Verification items for the finished model (mm, model axes). A direction names the side the tool comes from. Give positions to 0.01 mm unless a question says otherwise; leave off trailing zeros. Write each loop counter-clockwise with the first axis right and the second up, starting at its lowest first coordinate (ties: lowest second). Pieces come first, ordered by that corner, then holes. Notation, with made-up numbers: (81, 15) - (122, 15) arc R21 ccw to (122, 51) - close; hole circle Ø10 at (85, -22). An arc over 180 degrees is marked (long way). Put each result on its own line as item: value.
from build123d import *

# Parameters (mm, degrees)
F2_R     = 2
F3_DEPTH = 12.5
F5_R     = 2
F6_DEPTH = 25


with BuildPart() as f1:
    # F0 (on Top) → F1 (revolve)
    with BuildSketch(Plane.XY):
        with BuildLine():
            Line((32.238782, 5), (-36.118835, 5))
            ThreePointArc((-36.118835, 5), (-47.25717, 4.119532), (-58.118835, 1.5))
            ThreePointArc((-58.118835, 1.5), (-59.179495, 1.06066), (-59.618835, 0))
            Line((-59.618835, 0), (-58.118835, 0))
            Line((-58.118835, 0), (-36.118835, 0))
            Line((-36.118835, 0), (32.238782, 0))
            Line((32.238782, 0), (50.381165, 0))
            ThreePointArc((50.381165, 0), (41.648166, 3.727125), (32.238782, 5))
        make_face()
    revolve(axis=Axis((-7.075977, 0, 0), (1, 0, 0)))

    # F2 (on Front) → F3 (cut, symmetric)
    with BuildSketch(Plane.XZ):
        with Locations((30.381165, 0)):
            Circle(F2_R)
        with Locations((39.381165, 0)):
            Circle(F2_R)
    extrude(amount=F3_DEPTH, both=True, mode=Mode.SUBTRACT)

    # F5 (on offset) → F6 (cut)
    with BuildSketch(Plane.YZ.offset(30)):
        with Locations((5, 0)):
            Circle(F5_R)
        with Locations((-5, 0)):
            Circle(F5_R)
    extrude(amount=F6_DEPTH, mode=Mode.SUBTRACT)


solid = f1.part
Q1. Go/stop test with flat-tipped pins: pin 1 Ø2 at (y, z) = (1.5, -0.5) entering from +X; pin 2 Ø4 at (x, y) = (-41.5, -1.5) entering from +Z; pin 3 Ø6 at (x, y) = (25.5, 4) entering from -Z. Record where each tip stops, or that it passes through.
Answers follow:
pin 1: stops at x = 49.37
pin 2: stops at z = 4.89
pin 3: stops at z = -4.9
Q2. Section check A-A, the plane x = -23. Record the cut outline in (y, z), plus the area to 3 significant figures.
Answers follow:
outline: circle Ø10 at (0, 0)
area: 78.5 mm2
Q3. Set-up check for faces 4 (the face through (42, 3, 0)), 5 (the face through (28.383, -0.072, 0.088)), 6 (the face through (42, -3, 0)): record each of +Z, -Z, +X, -X, +Y, -Y from which the full face is reachable in a straight line by a thin tool's end or side.
Answers follow:
face 4: +X, +Y
face 5: +Y, -Y
face 6: +X, -Y
Q4. Release check for a two-part mould opening along Z. For faces 1 (the face through (35, -3, 0)), 2 (the face through (-2.42, -1.08, -4.88)), 3 (the face through (35, 3, 0)) record: released by +Z, released by -Z, zero draft, split by the parting line, or undercut.
Answers follow:
face 1: undercut
face 2: split by the parting line
face 3: undercut
Q5. Scan lines: line 1 along X through (y, z) = (-0.5, 0); line 2 along X through (y, z) = (-0.75, 0); line 3 along Y through (x, z) = (22.5, 4). Record each from-to range of solid material in increasing order.
Answers follow:
line 1: x = -59.53 to 28.38, 32.38 to 37.38, 41.38 to 49.52
line 2: x = -59.42 to 28.38, 32.38 to 37.38, 41.38 to 49.06
line 3: y = -3 to 3
